Check sheet for the modelled part. Datum: model origin and axes. Units: mm. A direction names the side the tool comes from. Round coordinates to 2 decimals unless told otherwise and drop trailing zeros. Write each loop counter-clockwise with the first axis right and the second up, starting at its lowest first coordinate (ties: lowest second). Pieces come first, ordered by that corner, then holes. Notation, with made-up numbers: M -30.5,-3 L 1.5,-3 A18 ccw 1.5,7 Z; hole C 57.25,29.25 d1. An arc over 180 degrees is marked long. Answer in a Markdown table with one row per item.
```python
from build123d import *

# Parameters (mm, degrees)
CUT_EXTRUDE_1_DEPTH = 2


with BuildPart() as part:
    # Sketch 1 → Revolve 1 (revolve)
    with BuildSketch(Plane(origin=(0, 0, 0), x_dir=(0, 0, -1), z_dir=(1, 0, 0)), mode=Mode.PRIVATE) as revolve_1_sk:
        Polygon((-4, 0), (-4, 3.2), (-3.7, 3.5), (0, 3.5), (0, 2), (49.5705, 2), (50, 1.5705), (50, 0), align=None)
    revolve(revolve_1_sk.sketch.rotate(Axis((0, 0, -50), (0, 0, 1)), 270), axis=Axis((0, 0, -50), (0, 0, 1)))

    # Sketch 2 → Cut-Extrude 1 (cut)
    with BuildSketch(Plane.XY.offset(4)):
        Polygon((-0.866025404, -1.5), (0.866025404, -1.5), (1.732050808, 0), (0.866025404, 1.5), (-0.866025404, 1.5), (-1.732050808, 0), align=None)
    extrude(amount=-CUT_EXTRUDE_1_DEPTH, mode=Mode.SUBTRACT)


solid = part.part
```
1. Scan lines: L1, parallel to Y at x = -1, z = -7; L2, parallel to Y at x = 0, z = -18; L3, parallel to Z at x = -3, y = 0.75. Record each from-to range of solid material in increasing order.
Found:
| item | result |
|---|---|
| L1 | y = -1.73 to 1.73 |
| L2 | y = -2 to 2 |
| L3 | z = 0 to 4 |
2. Section check A-A, the plane x = 0. Record the cut outline in (y, z).
Found:
| item | result |
|---|---|
| outline | M -3.5,0 L -2,0 L -2,-49.57 L -1.57,-50 L 1.57,-50 L 2,-49.57 L 2,0 L 3.5,0 L 3.5,3.7 L 3.2,4 L 1.5,4 L 1.5,2 L -1.5,2 L -1.5,4 L -3.2,4 L -3.5,3.7 Z |
3. Access from +Z, -Z, +X, -X, +Y, -Y to the whole of each face (thin tool, end or side, straight path). Record for faces 5 (the face through (1.5, 0.8, 4)), 6 (the face through (2, -2, 0)), 7 (the face through (-1.293, 0.76, 3.014)).
Found:
| item | result |
|---|---|
| face 5 | +Z, +X, -X, +Y, -Y |
| face 6 | -Z |
| face 7 | +Z |
4. Draft check along Y on faces 1 (the face through (-0.759, -3.417, 1.824)), 2 (the face through (0, 1.5, 3)), 3 (the face through (0, 0, -50)), 4 (the face through (1.293, -0.76, 3.014)). Enter one of: +Y half, -Y half, draft (parallel to the pull), parting line (faces both ways), or undercut.
Found:
| item | result |
|---|---|
| face 1 | parting line |
| face 2 | undercut |
| face 3 | draft |
| face 4 | undercut |
5. Go/stop test with flat-tipped pins: pin 1 (1.5 mm diameter, centred on x = 0, z = -23, fed in from -Y); pin 2 (3 mm diameter, centred on x = 2, y = -2.5, fed in from -Z); pin 3 (4 mm diameter, centred on y = 0, z = -3.5, fed in from -X). Record where each tip stops, or that it passes through.
Found:
| item | result |
|---|---|
| pin 1 | stops at y = -2 |
| pin 2 | stops at z = -49.87 |
| pin 3 | stops at x = -2 |
6. Section check B-B, the plane z = -19. Record the cut outline in (x, y).
Found:
| item | result |
|---|---|
| outline | C 0,0 d4 |
